Could you check a few things on this model? Use its own coordinates, in mm. A direction names the side the tool comes from. Coordinates: 2 decimals unless noted, no trailing zeros. One line per question, with ' | ' between items. Start each with the question number.
(1) Which directions (+Z, -Z, +X, -X, +Y, -Y) give clear straight access to the entire face, cutting with the end or side of a thin tool? Please do faces 5 (the face through (-185, 118.03, 0)), 6 (the face through (180.777, 103, 0)).
(2) If we mould it in two halves opening along Y, with no side actions, what happens to faces 1 (the face through (-15, 44, -10)), 2 (the face through (0, 34.825, 0)), 3 (the face through (-0.6, 59.03, -0.14)), 4 (the face through (0.8, 65.05, -0.14))? For each: pulls with the +Y half, pulls with the -Y half, needs draft (parallel to the pull), parting line crosses it, or undercut.
(3) I'm going to push flat-ended pins straight in: pin 1 Ø1.5 at (x, z) = (-92, -5.5) entering from +Y; pin 2 Ø4 at (x, z) = (39.5, -3) entering from -Y; pin 3 Ø3 at (x, z) = (-74.5, -8) entering from -Y. Where does each tip first touch, or does it pass through?
(4) If I drill on line 1 along X through (y, z) = (101.5, 6.5); line 2 along Y through (x, z) = (37, 4.5); line 3 along X through (y, z) = (68, -0.75), over which ranges is the centre line in solid material (lowest first)?
```python
from build123d import *

# Parameters (mm, degrees)
SKETCH_1_R               = 3.1
SKETCH_1_R_2             = 1.6
EXTRUDE_1_DEPTH          = 10
SKETCH_7_W               = 9.5
SKETCH_7_H               = 20
EXTRUDE_2_DEPTH          = 30
CUT_EXTRUDE_1_DEPTH      = 399.034023277
CUT_EXTRUDE_1_DEPTH_BACK = 399.034023277
SKETCH_8_R               = 2.55


with BuildPart() as part:
    # 草图1 → 凸台-拉伸1 (new, symmetric)
    # profile 1 of 3: a face of its own
    with BuildSketch(Plane.XY):
        with BuildLine():
            Line((-49.723400677, 34.824923839), (50.276599325, 34.824923839))
            add(Edge.make_bspline(
                [(50.276599325, 34.824923839), (124.566445362, 17.843319342), (95.555290462, -188.079366879), (170.787580761, -12.360236435)],
                knots=[0, 0, 0, 0, 1, 1, 1, 1], degree=3))
            ThreePointArc((170.787580761, -12.360236435), (0.276599325, 88.030011373), (-170.23438211, -12.360236435))
            add(Edge.make_bspline(
                [(-49.723400677, 34.824923839), (-124.01324671, 17.843319337), (-95.002091812, -188.079366877), (-170.23438211, -12.360236435)],
                knots=[0, 0, 0, 0, 1, 1, 1, 1], degree=3))
        make_face()
        with Locations((-62.62746254, 65.411358975)):
            Circle(SKETCH_1_R, mode=Mode.SUBTRACT)
        with Locations((-76.733019619, 56.414584056)):
            Circle(SKETCH_1_R_2, mode=Mode.SUBTRACT)
        with Locations((-89.723400674, 48.914584057)):
            Circle(SKETCH_1_R_2, mode=Mode.SUBTRACT)
        with Locations((-67.983019619, 41.25913949)):
            Circle(SKETCH_1_R_2, mode=Mode.SUBTRACT)
        with Locations((-80.973400674, 33.759139488)):
            Circle(SKETCH_1_R_2, mode=Mode.SUBTRACT)
        with Locations((0.276599325, 76.530011374)):
            Circle(SKETCH_1_R, mode=Mode.SUBTRACT)
        with Locations((0.276599325, 44.030011375)):
            Circle(SKETCH_1_R, mode=Mode.SUBTRACT)
        with Locations((63.180661188, 65.411358975)):
            Circle(SKETCH_1_R, mode=Mode.SUBTRACT)
        with Locations((77.286218268, 56.414584056)):
            Circle(SKETCH_1_R_2, mode=Mode.SUBTRACT)
        with Locations((90.276599325, 48.914584057)):
            Circle(SKETCH_1_R_2, mode=Mode.SUBTRACT)
        with Locations((81.526599324, 33.759139488)):
            Circle(SKETCH_1_R_2, mode=Mode.SUBTRACT)
        with Locations((68.536218267, 41.25913949)):
            Circle(SKETCH_1_R_2, mode=Mode.SUBTRACT)
        with BuildLine():
            ThreePointArc((-36.011685017, 54.574370317), (-0.091755893, 59.031248881), (35.839117979, 54.663483137))
            ThreePointArc((35.839117979, 54.663483137), (39.472360183, 56.849455003), (37.290649352, 60.485257494))
            ThreePointArc((37.290649352, 60.485257494), (0.276599325, 65.052037292), (-36.737450702, 60.485257494))
            ThreePointArc((-36.737450702, 60.485257494), (-38.986236568, 57.209141311), (-36.011685017, 54.574370317))
        make_face(mode=Mode.SUBTRACT)
    # profile 2 of 3: a face of its own
    with BuildSketch(Plane.XY):
        with BuildLine():
            add(Edge.make_bspline(
                [(-189.723400675, 88.030011373), (-189.61780162, 34.842552906), (-170.23438211, -12.360236435)],
                knots=[0, 0, 0, 0.9050572, 0.9050572, 0.9050572], degree=2))
            ThreePointArc((-170.23438211, -12.360236435), (-98.657970523, 61.068551265), (0.276599915, 88.030011373))
            Line((0.276599915, 88.030011373), (-189.723400675, 88.030011373))
        make_face()
    # profile 3 of 3: a face of its own
    with BuildSketch(Plane.XY):
        with BuildLine():
            ThreePointArc((0.276599915, 88.030011373), (99.211169681, 61.068550966), (170.787580761, -12.360236435))
            add(Edge.make_bspline(
                [(190.276599325, 88.030011373), (190.171000271, 34.842552906), (170.787580761, -12.360236435)],
                knots=[0, 0, 0, 0.9050572, 0.9050572, 0.9050572], degree=2))
            Line((190.276599325, 88.030011373), (0.276599915, 88.030011373))
        make_face()
    extrude(amount=EXTRUDE_1_DEPTH, both=True)

    # 草图7 → 凸台-拉伸2 (add)
    with BuildSketch(Plane(origin=(0, 88.030011373, 0), x_dir=(1, 0, 0), z_dir=(0, 1, 0))):
        with Locations((-184.973400675, 0)):
            Rectangle(SKETCH_7_W, SKETCH_7_H)
        with Locations((185.526599325, 0)):
            Rectangle(SKETCH_7_W, SKETCH_7_H)
    extrude(amount=EXTRUDE_2_DEPTH)

    # 草图8 → 切除-拉伸1 (cut, two sides: drawn at the far end of the back side and taken through both)
    with BuildSketch(Plane.ZY.offset(189.723400675).offset(-CUT_EXTRUDE_1_DEPTH_BACK)):
        with Locations((-4, 103.030011373)):
            Circle(SKETCH_8_R)
        with Locations((4, 103.030011373)):
            Circle(SKETCH_8_R)
    extrude(amount=CUT_EXTRUDE_1_DEPTH + CUT_EXTRUDE_1_DEPTH_BACK, mode=Mode.SUBTRACT)


solid = part.part
```
Checks:
1) face 5: +Z, -Z, +X, -X, +Y | face 6: +Z, -Z, +Y
2) face 1: needs draft | face 2: pulls with the -Y half | face 3: undercut | face 4: undercut
3) pin 1: stops at y = 88.03 | pin 2: stops at y = 34.82 | pin 3: stops at y = 17.45
4) line 1: x = -189.72 to -180.22, 180.78 to 190.28 | line 2: y = 34.82 to 54.61, 60.56 to 88.03 | line 3: x = -188.98 to -64.33, -60.92 to 61.48, 64.89 to 189.54
